Model file for the job. Use its own axes, mm. Face numbers are marked on the shaded views. A direction names the side the tool comes from. Round coordinates to 2 decimals unless told otherwise and drop trailing zeros. Order: outer loops, then holes, each group sorted by start corner. A loop starts at its lowest first (then second) coordinate and runs counter-clockwise, first axis right, second up. Notation, with made-up numbers: (81.25, 63.5) - (117.25, 63.5) arc R26 cw to (117.25, 102.5) - close; hole circle Ø3 at (-20, -15.5). An arc over 180 degrees is marked (long way). Answer as CSV lines item,"result". Start each with the question number.
1. 3-axis set-ups, long thin cutter, end or side, ignore diameter. For the marked faces 5 and 6: which of +Z, -Z, +X, -X, +Y, -Y reach the whole face in a straight line?
2. Band-saw the part on A-A on z = -13.5. List the corners of the cut face in (x, y).
3. Wall check: line 1 along Z through (x, y) = (45, 91); line 2 along X through (y, z) = (143, -27); line 3 along Y through (x, z) = (33, -14.5). Give the ranges that are in metal, low to high. Write a range as [from, to].
4. Band-saw the part on C-C on x = -55.5. List the corners of the cut face in (y, z), then the cut area to 3 significant figures.
5. Pin check, flat tips, straight feed: pin 1 Ø2 at (x, z) = (2, -33.5) entering from +Y; pin 2 Ø5 at (x, z) = (-19.5, 8) entering from +Y. Stop position of each tip, or through.
6. Pull direction X, two halves, no side cores. Call the marked faces 1, 2, 3 and 4: released by +X, released by -X, zero draft, split by the parting line, or undercut.
7. Band-saw the part on B-B on y = 159. List the corners of the cut face in (x, z), then the cut area to 3 significant figures.
```python
from build123d import *

# Parameters (mm, degrees)
SKETCH1_W           = 160
SKETCH1_H           = 80
BOSS_EXTRUDE1_DEPTH = 225
SKETCH2_W           = 150
SKETCH2_H           = 70
CUT_EXTRUDE1_DEPTH  = 220
SKETCH7_W           = 2
SKETCH7_H           = 120
BOSS_EXTRUDE2_DEPTH = 5
SKETCH8_W           = 2
SKETCH8_H           = 120
BOSS_EXTRUDE3_DEPTH = 5
SKETCH9_W           = 2
SKETCH9_H           = 120
BOSS_EXTRUDE4_DEPTH = 5
SKETCH10_W          = 2
SKETCH10_H          = 120
BOSS_EXTRUDE5_DEPTH = 5
SKETCH11_W          = 160
SKETCH11_H          = 80
SKETCH11_W_2        = 150
SKETCH11_H_2        = 70
CUT_EXTRUDE2_DEPTH  = 25


with BuildPart() as part:
    # Sketch1 → Boss-Extrude1 (new body)
    with BuildSketch(Plane(origin=(0, 0, 0), x_dir=(1, 0, 0), z_dir=(0, 1, 0))):
        Rectangle(SKETCH1_W, SKETCH1_H)
    extrude(amount=BOSS_EXTRUDE1_DEPTH)

    # Sketch2 → Cut-Extrude1 (cut)
    with BuildSketch(Plane(origin=(0, 225, 0), x_dir=(1, 0, 0), z_dir=(0, 1, 0))):
        Rectangle(SKETCH2_W, SKETCH2_H)
    extrude(amount=-CUT_EXTRUDE1_DEPTH, mode=Mode.SUBTRACT)

    # Sketch7 → Boss-Extrude2 (add)
    with BuildSketch(Plane(origin=(0, 0, 35), x_dir=(-1, 0, 0), z_dir=(0, 0, -1))):
        with Locations((-39.5, 65)):
            Rectangle(SKETCH7_W, SKETCH7_H)
        with Locations((-35.5, 65)):
            Rectangle(SKETCH7_W, SKETCH7_H)
        with Locations((-2, 65)):
            Rectangle(SKETCH7_W, SKETCH7_H)
        with Locations((2, 65)):
            Rectangle(SKETCH7_W, SKETCH7_H)
        with Locations((35.5, 65)):
            Rectangle(SKETCH7_W, SKETCH7_H)
        with Locations((39.5, 65)):
            Rectangle(SKETCH7_W, SKETCH7_H)
    extrude(amount=BOSS_EXTRUDE2_DEPTH)

    # Sketch8 → Boss-Extrude3 (add)
    with BuildSketch(Plane.XY.offset(-35)):
        with Locations((-39.5, 65)):
            Rectangle(SKETCH8_W, SKETCH8_H)
        with Locations((-35.5, 65)):
            Rectangle(SKETCH8_W, SKETCH8_H)
        with Locations((-2, 65)):
            Rectangle(SKETCH8_W, SKETCH8_H)
        with Locations((2, 65)):
            Rectangle(SKETCH8_W, SKETCH8_H)
        with Locations((35.5, 65)):
            Rectangle(SKETCH8_W, SKETCH8_H)
        with Locations((39.5, 65)):
            Rectangle(SKETCH8_W, SKETCH8_H)
    extrude(amount=BOSS_EXTRUDE3_DEPTH)

    # Sketch9 → Boss-Extrude4 (add)
    with BuildSketch(Plane(origin=(-75, 0, 0), x_dir=(0, 0, -1), z_dir=(1, 0, 0))):
        with Locations((-2, 65)):
            Rectangle(SKETCH9_W, SKETCH9_H)
        with Locations((2, 65)):
            Rectangle(SKETCH9_W, SKETCH9_H)
    extrude(amount=BOSS_EXTRUDE4_DEPTH)

    # Sketch10 → Boss-Extrude5 (add)
    with BuildSketch(Plane.ZY.offset(-75)):
        with Locations((-2, 65)):
            Rectangle(SKETCH10_W, SKETCH10_H)
        with Locations((2, 65)):
            Rectangle(SKETCH10_W, SKETCH10_H)
    extrude(amount=BOSS_EXTRUDE5_DEPTH)

    # Sketch11 → Cut-Extrude2 (cut)
    with BuildSketch(Plane(origin=(0, 225, 0), x_dir=(1, 0, 0), z_dir=(0, 1, 0))):
        Rectangle(SKETCH11_W, SKETCH11_H)
        Rectangle(SKETCH11_W_2, SKETCH11_H_2, mode=Mode.SUBTRACT)
    extrude(amount=-CUT_EXTRUDE2_DEPTH, mode=Mode.SUBTRACT)


solid = part.part
```
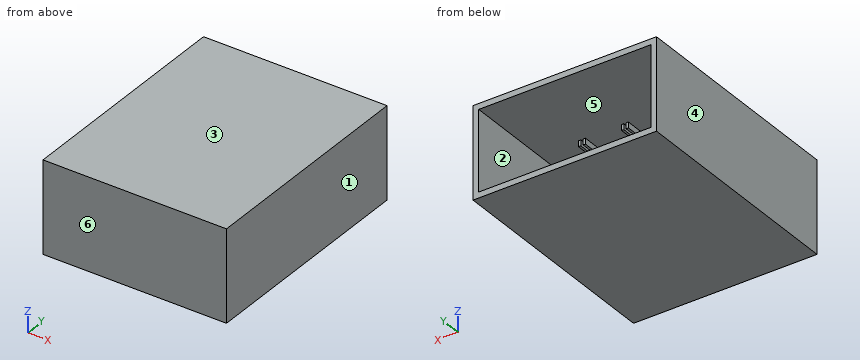
Reply:
1,face 5,"+Y"
1,face 6,"+Z, -Z, +X, -X, -Y"
2,outline,"(-80, 0) - (80, 0) - (80, 200) - (75, 200) - (75, 5) - (-75, 5) - (-75, 200) - (-80, 200) - close"
3,line 1,"z = [-40, -35], [35, 40]"
3,line 2,"x = [-80, -75], [75, 80]"
3,line 3,"y = [0, 5]"
4,outline,"(0, -40) - (200, -40) - (200, -35) - (5, -35) - (5, 35) - (200, 35) - (200, 40) - (0, 40) - close"
4,area,"2,350 mm2"
5,pin 1,"stops at y = 125"
5,pin 2,"stops at y = 5"
6,face 1,"released by +X"
6,face 2,"undercut"
6,face 3,"zero draft"
6,face 4,"released by -X"
7,outline,"(-80, -40) - (80, -40) - (80, 40) - (-80, 40) - close; hole (-75, -35) - (75, -35) - (75, 35) - (-75, 35) - close"
7,area,"2,300 mm2"
